from build123d import *

# Parameters (mm, degrees)
SKETCH1_W           = 132
SKETCH1_H           = 87
BOSS_EXTRUDE1_DEPTH = 1.5
SKETCH2_W           = 80
SKETCH2_H           = 55
BOSS_EXTRUDE2_DEPTH = 2
SKETCH3_W           = 77
SKETCH3_H           = 52
CUT_EXTRUDE1_DEPTH  = 2
CUT_EXTRUDE2_REACH  = 3.5
SKETCH4_W           = 70
SKETCH4_H           = 45
SKETCH5_W           = 1.5
SKETCH5_H           = 41
SKETCH5_W_2         = 66
SKETCH5_H_2         = 1.5
CUT_EXTRUDE3_DEPTH  = 2
CUT_EXTRUDE4_DEPTH  = 1.5


with BuildPart() as part:
    # Sketch1 → Boss-Extrude1 (new body)
    with BuildSketch(Plane(origin=(0, 0, 0), x_dir=(1, 0, 0), z_dir=(0, 1, 0))):
        Rectangle(SKETCH1_W, SKETCH1_H)
    extrude(amount=BOSS_EXTRUDE1_DEPTH)

    # Sketch2 → Boss-Extrude2 (add)
    with BuildSketch(Plane(origin=(0, 1.5, 0), x_dir=(1, 0, 0), z_dir=(0, 1, 0))):
        Rectangle(SKETCH2_W, SKETCH2_H)
    extrude(amount=BOSS_EXTRUDE2_DEPTH)

    # Sketch3 → Cut-Extrude1 (cut)
    with BuildSketch(Plane(origin=(0, 3.5, 0), x_dir=(1, 0, 0), z_dir=(0, 1, 0))):
        Rectangle(SKETCH3_W, SKETCH3_H)
    extrude(amount=-CUT_EXTRUDE1_DEPTH, mode=Mode.SUBTRACT)

    # Sketch4 → Cut-Extrude2 (cut, up to next)
    with BuildSketch(Plane(origin=(0, 1.5, 0), x_dir=(1, 0, 0), z_dir=(0, 1, 0)), mode=Mode.PRIVATE) as cut_extrude2_sk1:
        Rectangle(SKETCH4_W, SKETCH4_H)
    cut_extrude2_tool1 = extrude(cut_extrude2_sk1.sketch, amount=-CUT_EXTRUDE2_REACH, mode=Mode.PRIVATE) & part.part
    add(cut_extrude2_tool1.solids().sort_by_distance((0, 1.5, 0))[0], mode=Mode.SUBTRACT)

    # Sketch5 → Cut-Extrude3 (cut)
    with BuildSketch(Plane(origin=(0, 3.5, 0), x_dir=(1, 0, 0), z_dir=(0, 1, 0))):
        with Locations((-39.25, 0)):
            Rectangle(SKETCH5_W, SKETCH5_H)
        with Locations((39.25, 0)):
            Rectangle(SKETCH5_W, SKETCH5_H)
        with Locations((0, 26.75)):
            Rectangle(SKETCH5_W_2, SKETCH5_H_2)
        with Locations((0, -26.75)):
            Rectangle(SKETCH5_W_2, SKETCH5_H_2)
    extrude(amount=-CUT_EXTRUDE3_DEPTH, mode=Mode.SUBTRACT)

    # Sketch6 → Cut-Extrude4 (cut)
    with BuildSketch(Plane(origin=(0, 1.5, 0), x_dir=(1, 0, 0), z_dir=(0, 1, 0))):
        with BuildLine():
            Line((-8, 43.5), (8, 43.5))
            ThreePointArc((8, 43.5), (0, 35.5), (-8, 43.5))
        make_face()
    extrude(amount=-CUT_EXTRUDE4_DEPTH, mode=Mode.SUBTRACT)


solid = part.part
Build history of the part. All positions in model axes, mm. Coordinates: 2 decimals unless noted, no trailing zeros. Order: outer loops, then holes, each group sorted by start corner. A loop starts at its lowest first (then second) coordinate and runs counter-clockwise, first axis right, second up. Notation, with made-up numbers: (2, -12.75) - (48, -12.75) arc R24 ccw to (48, 13.25) - close; hole circle Ø7 at (80, 52). An arc over 180 degrees is marked (long way). Write item = value, one per line. Start each with the question number.
1) Two-plate mould, pull along X, no slides. Class faces 1 (the face through (0.176, 0.76, -35.502)), 2 (the face through (-1, 0, 28)): pulls with the +X half, pulls with the -X half, needs draft (parallel to the pull), parting line crosses it, or undercut.
2) Wall check: line 1 along Z through (x, y) = (11.5, 1); line 2 along X through (y, z) = (1.25, 0.5); line 3 along Z through (x, y) = (34.5, 2.5). Give the ranges that are in metal, low to high. Write a range as from..to.
3) Saw through at A-A on x = 0. Write the cut outline in (y, z), then the cut area to 3 significant figures.
4) Saw through at B-B on z = -2. Write the cut outline in (x, y).
5) Flat gauge pins, fed straight in: pin 1 Ø1 at (y, z) = (3, 24) entering from +X; pin 2 Ø1.6 at (x, y) = (-35, 2.5) entering from -Z; pin 3 Ø0.6 at (y, z) = (2.5, 24.5) entering from -X. Where does each tip first touch, or does it go through?
6) Saw through at C-C on y = 2.65. Write the cut outline in (x, z).
7) Saw through at D-D on z = -33.5. Write the cut outline in (x, y), then the cut area to 3 significant figures.
From the geometry:
q1.face_1 = undercut
q1.face_2 = needs draft
q2.line_1 = -43.5..-22.5, 22.5..43.5
q2.line_2 = -66..-35, 35..66
q2.line_3 = -27.5..-26, 26..27.5
q3.outline = (0, -35.5) - (1.5, -35.5) - (1.5, -22.5) - (0, -22.5) - close; (0, 22.5) - (1.5, 22.5) - (1.5, 43.5) - (0, 43.5) - close
q3.area = 51.0 mm^2
q4.outline = (-66, 0) - (-35, 0) - (-35, 1.5) - (-66, 1.5) - close; (35, 0) - (66, 0) - (66, 1.5) - (35, 1.5) - close
q5.pin_1 = 40
q5.pin_2 = -27.5
q5.pin_3 = -40
q6.outline = (-40, -27.5) - (-33, -27.5) - (-33, -26) - (-38.5, -26) - (-38.5, -20.5) - (-40, -20.5) - close; (-40, 20.5) - (-38.5, 20.5) - (-38.5, 26) - (-33, 26) - (-33, 27.5) - (-40, 27.5) - close; (33, -27.5) - (40, -27.5) - (40, -20.5) - (38.5, -20.5) - (38.5, -26) - (33, -26) - close; (33, 26) - (38.5, 26) - (38.5, 20.5) - (40, 20.5) - (40, 27.5) - (33, 27.5) - close
q7.outline = (-66, 0) - (66, 0) - (66, 1.5) - (-66, 1.5) - close
q7.area = 198 mm^2
